```python
from build123d import *

# Parameters (mm, degrees)
F0_R     = 15.5
F1_DEPTH = 10
F2_R     = 14
F3_DEPTH = 25
F4_R     = 14.25
F5_DEPTH = 8


with BuildPart() as f1:
    # F0 (on Top) → F1 (new body)
    with BuildSketch(Plane.XY):
        Circle(F0_R)
    extrude(amount=F1_DEPTH)

    # F2 (on Top) → F3 (cut)
    with BuildSketch(Plane.XY):
        Circle(F2_R)
    extrude(amount=F3_DEPTH, mode=Mode.SUBTRACT)

    # F4 (on Top) → F5 (cut)
    with BuildSketch(Plane.XY):
        Circle(F4_R)
    extrude(amount=F5_DEPTH, mode=Mode.SUBTRACT)


solid = f1.part
```
Geometry: final body of the model. Coordinates: model frame, mm. Coordinates: 2 decimals unless noted, no trailing zeros. Order: outer loops, then holes, each group sorted by start corner. A loop starts at its lowest first (then second) coordinate and runs counter-clockwise, first axis right, second up. Notation, with made-up numbers: M 68.5,43 L 96.5,43 A25 ccw 96.5,72 Z; hole C 75,-23.5 d7. An arc over 180 degrees is marked long. Answer in a Markdown table with one row per item. Add a question column.
Q1. Section query C-C on z = 6.5. Return the cut outline in (x, y), and give its area (3 significant figures).
Q2. Line query: L1, parallel to Y at x = 0, z = 8.4; L2, parallel to Y at x = 0, z = 5; L3, parallel to X at y = 10.5, z = 6.75. Output: solid intervals per line, ascending.
Q3. Mould query, pull axis X, two halves, no side actions, for faces 1 (the cylindrical face through (13.163, -5.458, 3.944)), 2 (the flat face through (13, -7, 0)), 3 (the cylindrical face through (-2.018, 15.368, 4.93)), 4 (the cylindrical face through (12.932, -5.362, 8.986)). Classes: released by +X, released by -X, zero draft, split by the parting line, or undercut.
Q4. Section query A-A on x = 0. Return the cut outline in (y, z), and give its area (3 significant figures).
Q5. Contact query for flat-ended pins moving along their axis: P1, Ø1, axis at y = -9.5, z = 1.5, coming from the -X side; P2, Ø1, axis at y = -2, z = 6.5, coming from the +X side; P3, Ø6, axis at x = 11, z = 6.5, coming from the +Y side. Output: stop coordinate, or through.
Completed:
| question | item | result |
|---|---|---|
| 1 | outline | C 0,0 d31; hole C 0,0 d28.5 |
| 1 | area | 117 mm2 |
| 2 | L1 | y = -15.5 to -14, 14 to 15.5 |
| 2 | L2 | y = -15.5 to -14.25, 14.25 to 15.5 |
| 2 | L3 | x = -11.4 to -9.63, 9.63 to 11.4 |
| 3 | face 1 | undercut |
| 3 | face 2 | zero draft |
| 3 | face 3 | split by the parting line |
| 3 | face 4 | undercut |
| 4 | outline | M -15.5,0 L -14.25,0 L -14.25,8 L -14,8 L -14,10 L -15.5,10 Z; M 14,8 L 14.25,8 L 14.25,0 L 15.5,0 L 15.5,10 L 14,10 Z |
| 4 | area | 26.0 mm2 |
| 5 | P1 | stops at x = -12.62 |
| 5 | P2 | stops at x = 15.43 |
| 5 | P3 | stops at y = 13.28 |
